Source: CAD feature listing. Evaluate the final solid. Frame: model axes, mm. A direction names the side the tool comes from. Give positions to 0.01 mm unless a question says otherwise; leave off trailing zeros.
```python
from build123d import *

# Parameters (mm, degrees)
ESQUISSE1_W                  = 250
ESQUISSE1_H                  = 890
BOSS_EXTRU_1_DEPTH           = 180
ESQUISSE2_W                  = 250
ESQUISSE2_H                  = 100
ENL_V_MAT_EXTRU_1_DEPTH      = 1258.497514908
ENL_V_MAT_EXTRU_2_DEPTH      = 1325.726386844
ENL_V_MAT_EXTRU_2_DEPTH_BACK = 1325.726386844
ESQUISSE3_W                  = 100
ESQUISSE3_H                  = 230
ESQUISSE3_H_2                = 970
BOSS_EXTRU_2_REACH           = 1331.248
ESQUISSE6_W                  = 40
ESQUISSE6_H                  = 40
COQUE1_START                 = 4
COQUE1_OUTLINE_W             = 258
COQUE1_OUTLINE_H             = 898
COQUE1_DEPTH                 = 32
COQUE1_START_2               = 144
COQUE1_2_OUTLINE_W           = 258
COQUE1_2_OUTLINE_H           = 898
COQUE1_2_DEPTH               = 32
COQUE1_START_3               = 36
COQUE1_3_OUTLINE_W           = 32
COQUE1_3_OUTLINE_H           = 72
COQUE1_3_OUTLINE_H_2         = 32
COQUE1_3_DEPTH               = 108
ESQUISSE8_R                  = 15
ENL_V_MAT_EXTRU_5_DEPTH      = 1335.053971922


# Read off the part's stored shape, not the designer's step: Coque1
with BuildPart() as part:
    # Esquisse1 → Boss.-Extru.1 (new body)
    with BuildSketch(Plane.XY):
        Polygon((0, -80), (0, -1200), (40, -1280), (290, -1280), (330, -1200), (330, -80), (290, -80), (290, -230), (40, -230), (40, -80), align=None)
        with Locations((165, -755)):
            Rectangle(ESQUISSE1_W, ESQUISSE1_H, mode=Mode.SUBTRACT)
    extrude(amount=BOSS_EXTRU_1_DEPTH)

    # Esquisse2 → Enlèv. mat.-Extru.1 (cut, through all)
    with BuildSketch(Plane(origin=(0, -80, 0), x_dir=(1, 0, 0), z_dir=(0, 1, 0))):
        with Locations((165, -90)):
            Rectangle(ESQUISSE2_W, ESQUISSE2_H)
    extrude(amount=-ENL_V_MAT_EXTRU_1_DEPTH, mode=Mode.SUBTRACT)

    # Esquisse3 → Enlèv. mat.-Extru.2 (cut, two sides: drawn at the far end of the back side and taken through both)
    with BuildSketch(Plane.ZY.offset(-290).offset(-ENL_V_MAT_EXTRU_2_DEPTH_BACK)):
        with Locations((90, -115)):
            Rectangle(ESQUISSE3_W, ESQUISSE3_H)
        with Locations((90, -795)):
            Rectangle(ESQUISSE3_W, ESQUISSE3_H_2)
    extrude(amount=ENL_V_MAT_EXTRU_2_DEPTH + ENL_V_MAT_EXTRU_2_DEPTH_BACK, mode=Mode.SUBTRACT)

    # Esquisse6 → Boss.-Extru.2 (add, up to next)
    with BuildSketch(Plane(origin=(0, 0, 140), x_dir=(-1, 0, 0), z_dir=(0, 0, -1)), mode=Mode.PRIVATE) as boss_extru_2_sk1:
        with Locations((-310, -860)):
            Rectangle(ESQUISSE6_W, ESQUISSE6_H)
    boss_extru_2_tool1 = extrude(boss_extru_2_sk1.sketch, amount=BOSS_EXTRU_2_REACH, mode=Mode.PRIVATE) - part.part
    # Esquisse6 → Boss.-Extru.2 (add, up to next)
    with BuildSketch(Plane(origin=(0, 0, 140), x_dir=(-1, 0, 0), z_dir=(0, 0, -1)), mode=Mode.PRIVATE) as boss_extru_2_sk2:
        with Locations((-20, -860)):
            Rectangle(ESQUISSE6_W, ESQUISSE6_H)
    boss_extru_2_tool2 = extrude(boss_extru_2_sk2.sketch, amount=BOSS_EXTRU_2_REACH, mode=Mode.PRIVATE) - part.part
    add(boss_extru_2_tool1.solids().sort_by_distance((310, -860, 140))[0])
    add(boss_extru_2_tool2.solids().sort_by_distance((20, -860, 140))[0])

    # Coque1 outline → Coque1 (cut)
    with BuildSketch(Plane.XY.offset(COQUE1_START)):
        Polygon((294, -234), (36, -234), (36, -84), (4, -84), (4, -1199.05572809), (42.472135955, -1276), (287.527864045, -1276), (326, -1199.05572809), (326, -84), (294, -84), align=None)
        with Locations((165, -755)):
            Rectangle(COQUE1_OUTLINE_W, COQUE1_OUTLINE_H, mode=Mode.SUBTRACT)
    extrude(amount=COQUE1_DEPTH, mode=Mode.SUBTRACT)

    # Coque1 2 outline → Coque1 2 (cut)
    with BuildSketch(Plane.XY.offset(COQUE1_START_2)):
        Polygon((294, -234), (36, -234), (36, -84), (4, -84), (4, -1199.05572809), (42.472135955, -1276), (287.527864045, -1276), (326, -1199.05572809), (326, -84), (294, -84), align=None)
        with Locations((165, -755)):
            Rectangle(COQUE1_2_OUTLINE_W, COQUE1_2_OUTLINE_H, mode=Mode.SUBTRACT)
    extrude(amount=COQUE1_2_DEPTH, mode=Mode.SUBTRACT)

    # Coque1 3 outline → Coque1 3 (cut)
    with BuildSketch(Plane.XY.offset(COQUE1_START_3)):
        with Locations((310, -270)):
            Rectangle(COQUE1_3_OUTLINE_W, COQUE1_3_OUTLINE_H)
        with Locations((310, -860)):
            Rectangle(COQUE1_3_OUTLINE_W, COQUE1_3_OUTLINE_H_2)
        with Locations((20, -270)):
            Rectangle(COQUE1_3_OUTLINE_W, COQUE1_3_OUTLINE_H)
        with Locations((20, -860)):
            Rectangle(COQUE1_3_OUTLINE_W, COQUE1_3_OUTLINE_H_2)
    extrude(amount=COQUE1_3_DEPTH, mode=Mode.SUBTRACT)

    # Esquisse8 → Enlèv. mat.-Extru.5 (cut, through all)
    with BuildSketch(Plane(origin=(0, 0, 0), x_dir=(-1, 0, 0), z_dir=(0, 0, -1))):
        with Locations((-240, -1240)):
            Circle(ESQUISSE8_R)
    extrude(amount=-ENL_V_MAT_EXTRU_5_DEPTH, mode=Mode.SUBTRACT)


solid = part.part
```
1) Material intervals for L1, parallel to Z at x = 160, y = -287.5; L2, parallel to Y at x = 223, z = 144.5; L3, parallel to Y at x = 240, z = 143.1, sorted ascending.
Report:
L1: z = 0 to 4, 36 to 40, 140 to 144, 176 to 180
L2: y = -1280 to -1276, -1204 to -1200, -310 to -306, -234 to -230
L3: y = -1280 to -1255, -1225 to -1200, -310 to -230
2) Draft query along Z for faces 1 (the flat face through (20, -80, 160)), 2 (the flat face through (36, -761, 146)). Return one class per face: +Z half, -Z half, draft (parallel to the pull), parting line (faces both ways), or undercut.
Report:
face 1: draft
face 2: undercut
3) Pin query (flat end, axial travel): pin 1 (9.5 mm diameter, centred on x = 116, z = 27, fed in from +Y); pin 2 (12 mm diameter, centred on x = 313.5, z = 96, fed in from -Y). Return the tip coordinate at first contact, or that it passes through.
Report:
pin 1: stops at y = -230
pin 2: stops at y = -880
4) Reachability of faces 3 (the flat face through (310, -80, 160)), 4 (the flat face through (40, -271, 89)), 5 (the flat face through (167, -230, 20)), 6 (the flat face through (310, -571, 144)) from +Z, -Z, +X, -X, +Y, -Y: full face, straight path, thin tool, end or side. Return the list, or none.
Report:
face 3: +Z, -Z, +X, -X, +Y
face 4: +Y, -Y
face 5: +Z, -Z, +Y
face 6: none
5) Section query A-A, the plane y = -394. Count the separate pieces of the cut face and the enclosed holes in it, and give its area (3 significant figures).
Report:
separate pieces: 4
enclosed holes: 4
area: 2,300 mm2
